Can you work these out from the model? Positions are in its coordinate system, mm. A direction names the side the tool comes from. Give positions to 0.01 mm unless a question says otherwise; leave off trailing zeros. Order: outer loops, then holes, each group sorted by start corner. A loop starts at its lowest first (then second) coordinate and runs counter-clockwise, first axis right, second up. Notation, with made-up numbers: M 54.5,64 L 103.5,64 A32 ccw 103.5,96 Z; hole C 25,80.25 d10. An arc over 180 degrees is marked long. Answer as a JSON object with one key per item and string values.
```python
from build123d import *

# Parameters (mm, degrees)
F0_W        = 25
F0_H        = 30
F1_DEPTH    = 2
F2_R        = 1.5
F3_DEPTH    = 2.001
F4_W        = 1
F4_H        = 6.1
F5_DEPTH    = 0.9
F6_T1_DEPTH = 53.4336597593
F7_R        = 7


# Not quite as in the source:
# - a fillet or chamfer that OpenCascade refuses, or shapes differently, is made with other operations: its cross-section is extruded or revolved along the edge and cut away or added


with BuildPart() as f1:
    # F0 (on Top) → F1 (new body)
    with BuildSketch(Plane.XY):
        Rectangle(F0_W, F0_H)
    extrude(amount=F1_DEPTH)

    # F2 (on face) → F3 (cut, through all)
    with BuildSketch(Plane.XY.offset(2)):
        with Locations((-2, -12)):
            Circle(F2_R)
        with Locations((4.5, -1.5)):
            Circle(F2_R)
        with Locations((4.5, 8.5)):
            Circle(F2_R)
    extrude(amount=-F3_DEPTH, mode=Mode.SUBTRACT)

    # F4 (on face) → F5 (cut)
    with BuildSketch(Plane(origin=(0, 0, 0), x_dir=(1, 0, 0), z_dir=(0, 0, -1))):
        with Locations((11.6, -3.051)):
            Rectangle(F4_W, F4_H)
        with Locations((9.6, -3.051)):
            Rectangle(F4_W, F4_H)
        with Locations((7.6, -3.051)):
            Rectangle(F4_W, F4_H)
        with Locations((5.6, -3.051)):
            Rectangle(F4_W, F4_H)
        with Locations((3.6, -3.051)):
            Rectangle(F4_W, F4_H)
        with Locations((1.6, -3.051)):
            Rectangle(F4_W, F4_H)
        with Locations((-0.4, -3.051)):
            Rectangle(F4_W, F4_H)
        with Locations((-2.4, -3.051)):
            Rectangle(F4_W, F4_H)
        with Locations((-4.4, -3.051)):
            Rectangle(F4_W, F4_H)
        with Locations((-6.4, -3.051)):
            Rectangle(F4_W, F4_H)
        with Locations((-8.4, -3.051)):
            Rectangle(F4_W, F4_H)
        with Locations((-10.4, -3.051)):
            Rectangle(F4_W, F4_H)
        with Locations((-12.4, -3.051)):
            Rectangle(F4_W, F4_H)
    extrude(amount=-F5_DEPTH, mode=Mode.SUBTRACT)

    # F6: chamfer of 10 on 1 edges, made by hand

    # F6_s2 → F6_t1 (cut)
    with BuildSketch(Plane.XY.offset(-25.7168298797)):
        Polygon((-12.5, 5), (-2.5, 15), (-12.5, 15), align=None)
    extrude(amount=F6_T1_DEPTH, mode=Mode.SUBTRACT)

    # F7
    f7_edges = [f1.edges().sort_by_distance(p)[0] for p in [
        (-12.5, 5, 1.45),
        (-2.5, 15, 1),
        (12.5, 15, 1),
    ]]
    fillet(f7_edges, radius=F7_R)


solid = f1.part
```
1) I need wall thicknesses on L1, parallel to Y at x = 4.5, z = 0.5; L2, parallel to Y at x = 5.75, z = 0.15; L3, parallel to Y at x = -2.75, z = 0.2. Which ranges of each line are inside material? Lowest first, please.
Results found:
{"L1": "y = -15 to -3, 0 to 7, 10 to 15", "L2": "y = -15 to -2.33, -0.67 to 0, 6.1 to 7.67, 9.33 to 15", "L3": "y = -15 to -13.3, -10.7 to 0, 6.1 to 14.25"}
2) I want a section at D-D on x = 8.5. Write out the boundary of the cut face in (y, z), and give its area (3 significant figures).
Results found:
{"outline": "M -15,0 L 14.32,0 L 14.32,2 L -15,2 Z", "area": "58.6 mm²"}
3) I want a section at A-A on y = -1.5. Write out the boundary of the cut face in (x, z), and give its area (3 significant figures).
Results found:
{"outline": "M -12.5,0 L 3,0 L 3,2 L -12.5,2 Z; M 6,0 L 12.5,0 L 12.5,2 L 6,2 Z", "area": "44.0 mm²"}
4) I want a section at C-C on y = 8.5. Write out the boundary of the cut face in (x, z), and give its area (3 significant figures).
Results found:
{"outline": "M -9,0 L 3,0 L 3,2 L -9,2 Z; M 6,0 L 12.48,0 L 12.48,2 L 6,2 Z", "area": "37.0 mm²"}
5) I'm going to push flat-ended pins straight in: pin 1 Ø1 at (x, z) = (11.5, 0.5) entering from +Y; pin 2 Ø0.7 at (x, z) = (-6.5, 0.5) entering from +Y; pin 3 Ø0.5 at (x, y) = (-4.5, 4.5) entering from -Z. Where does each tip first touch, or does it pass through?
Results found:
{"pin 1": "stops at y = 12.33", "pin 2": "stops at y = 11.35", "pin 3": "stops at z = 0.9"}
6) I want a section at B-B on x = 4.5. Write out the boundary of the cut face in (y, z), and give its area (3 significant figures).
Results found:
{"outline": "M -15,0 L -3,0 L -3,2 L -15,2 Z; M 0,0 L 7,0 L 7,2 L 0,2 Z; M 10,0 L 15,0 L 15,2 L 10,2 Z", "area": "48.0 mm²"}
7) For faces 1 (the face through (12.1, 3.1, 0.4)), 2 (the face through (-11.9, 2.5, 0.4)), which set-ups out of +Z, -Z, +X, -X, +Y, -Y let a thin tool reach every point of the face, with its end or its side?
Results found:
{"face 1": "-Z", "face 2": "-Z, -X, +Y"}
